```python
from build123d import *

# Parameters (mm, degrees)
F0_W     = 0.8
F0_H     = 36.4
F0_W_2   = 8.8
F0_H_2   = 1.5
F1_DEPTH = 2
F2_DEPTH = 10
F3_DEPTH = 4.15
F0_H_3   = 3.6
F4_DEPTH = 2
F5_W     = 1.5
F5_H     = 2.85
F6_DEPTH = 8.8
F0_W_3   = 28.8
F0_H_4   = 1.2
F7_DEPTH = 10


with BuildPart() as f1:
    # F0 (on Top) → F1 (new body)
    with BuildSketch(Plane.XY):
        Polygon((-15.506923, -17.20208), (-15.506923, 31.19792), (-7.006923, 31.19792), (-7.006923, 32.69792), (-17.006923, 32.69792), (-17.006923, -18.70208), (11.793077, -18.70208), (11.793077, 32.69792), (1.793077, 32.69792), (1.793077, 31.19792), (10.293077, 31.19792), (10.293077, -17.20208), align=None)
        Polygon((-7.006923, 31.19792), (-15.506923, 31.19792), (-15.506923, -17.20208), (10.293077, -17.20208), (10.293077, 31.19792), (1.793077, 31.19792), align=None)
        with Locations((-13.956923, 6.99792)):
            Rectangle(F0_W, F0_H, mode=Mode.SUBTRACT)
        Polygon((8.343077, -11.20208), (8.343077, 21.59792), (7.483077, 21.59792), (7.483077, 26.77792), (8.743077, 26.77792), (10.003077, 26.77792), (10.003077, 21.59792), (9.143077, 21.59792), (9.143077, -11.20208), align=None, mode=Mode.SUBTRACT)
        with Locations((-2.606923, 31.94792)):
            Rectangle(F0_W_2, F0_H_2)
    extrude(amount=-F1_DEPTH)

    # F0 (on Top) → F2 (join)
    with BuildSketch(Plane.XY):
        Polygon((-15.506923, -17.20208), (-15.506923, 31.19792), (-7.006923, 31.19792), (-7.006923, 32.69792), (-17.006923, 32.69792), (-17.006923, -18.70208), (11.793077, -18.70208), (11.793077, 32.69792), (1.793077, 32.69792), (1.793077, 31.19792), (10.293077, 31.19792), (10.293077, -17.20208), align=None)
    extrude(amount=F2_DEPTH)

    # F0 (on Top) → F3 (join)
    with BuildSketch(Plane.XY):
        with Locations((-2.606923, 31.94792)):
            Rectangle(F0_W_2, F0_H_2)
    extrude(amount=F3_DEPTH)

    # F0 (on Top) → F4 (cut)
    with BuildSketch(Plane.XY):
        with Locations((-13.956923, 6.99792)):
            Rectangle(F0_W, F0_H)
        with Locations((8.743077, 23.39792)):
            Rectangle(F0_W, F0_H_3)
    extrude(amount=-F4_DEPTH, mode=Mode.SUBTRACT)

    # F5 (on face) → F6 (join)
    with BuildSketch(Plane.YZ.offset(-7.006923)):
        with Locations((31.94792, 8.575)):
            Rectangle(F5_W, F5_H)
    extrude(amount=F6_DEPTH)

    # F0 (on Top) → F7 (join)
    with BuildSketch(Plane.XY):
        with Locations((-2.606923, -19.30208)):
            Rectangle(F0_W_3, F0_H_4)
    extrude(amount=F7_DEPTH)


solid = f1.part
```
The model under review builds one solid part; all positions refer to its coordinate system, in mm. A direction names the side the tool comes from. Round coordinates to 2 decimals unless told otherwise and drop trailing zeros. Write each loop counter-clockwise with the first axis right and the second up, starting at its lowest first coordinate (ties: lowest second). Pieces come first, ordered by that corner, then holes. Notation, with made-up numbers: (71.5, 10) - (75.5, 10) arc R21 ccw to (75.5, 17) - close; hole circle Ø9 at (-18, 25). An arc over 180 degrees is marked (long way). Answer as CSV lines item,"result". Start each with the question number.
(1) We need section B-B on x = -2. State the section outline as (y, z) points.
(2) Draft analysis for pull direction Y (two halves, no side actions). For faces 6 (the flat face through (-3, -19, 0)), 7 (the flat face through (-3, -18.702, -1)), 8 (the flat face through (9, 26.778, -1)), state which applies: pulls with the +Y half, pulls with the -Y half, needs draft (parallel to the pull), parting line crosses it, or undercut.
(3) We need section A-A on y = -10. State the section outline as (x, z) points, plus the area to 3 significant figures.
(4) For faces 1 (the flat face through (-3, 32, 4.15)), 2 (the flat face through (-16.5, 6.5, 10)), 3 (the flat face through (-17.007, 6, 4)), 4 (the flat face through (-14.357, 7, -1)), 5 (the flat face through (-3, 31.198, 4)), list the 3-axis set-ups (+Z, -Z, +X, -X, +Y, -Y) from which the entire face can be reached by the end or side of a thin tool; tool diameter is ignored.
(5) For pin 1 Ø1 at (x, z) = (0.5, 5) entering from +Y; pin 2 Ø6 at (x, y) = (-7.5, -4.5) entering from +Z; pin 3 Ø1.3 at (x, y) = (-5.5, -19.5) entering from -Z, all flat-tipped, find the tip position at first contact; note any pin that passes through.
(6) To check wall thickness, follow line 1 (X direction, y = 21.5, z = -1.5); line 2 (Y direction, x = -9, z = 0.25); line 3 (X direction, y = -7.5, z = 7.5). State the ranges of each line that lie inside material, in increasing order.
(7) We need section D-D on y = -16. State the section outline as (x, z) points, plus the area to 3 significant figures.
(8) We need section C-C on z = 3. State the section outline as (x, y) points.
Worked answers:
1,outline,"(-19.9, 0) - (-18.7, 0) - (-18.7, -2) - (32.7, -2) - (32.7, 4.15) - (31.2, 4.15) - (31.2, 0) - (-17.2, 0) - (-17.2, 10) - (-19.9, 10) - close; (31.2, 7.15) - (32.7, 7.15) - (32.7, 10) - (31.2, 10) - close"
2,face 6,"needs draft"
2,face 7,"pulls with the -Y half"
2,face 8,"undercut"
3,outline,"(-17.01, -2) - (-14.36, -2) - (-14.36, 0) - (-15.51, 0) - (-15.51, 10) - (-17.01, 10) - close; (-13.56, -2) - (8.34, -2) - (8.34, 0) - (-13.56, 0) - close; (9.14, -2) - (11.79, -2) - (11.79, 10) - (10.29, 10) - (10.29, 0) - (9.14, 0) - close"
3,area,"84.4 mm²"
4,face 1,"+Y"
4,face 2,"+Z, +X, -X, +Y, -Y"
4,face 3,"+Z, -Z, -X, +Y, -Y"
4,face 4,"+Z, -Z"
4,face 5,"+Z"
5,pin 1,"y = -17.2"
5,pin 2,"z = 0"
5,pin 3,"z = 0"
6,line 1,"-17.01 to -14.36, -13.56 to 8.34, 9.14 to 11.79"
6,line 2,"-19.9 to -17.2, 31.2 to 32.7"
6,line 3,"-17.01 to -15.51, 10.29 to 11.79"
7,outline,"(-17.01, -2) - (11.79, -2) - (11.79, 10) - (10.29, 10) - (10.29, 0) - (-15.51, 0) - (-15.51, 10) - (-17.01, 10) - close"
7,area,"87.6 mm²"
8,outline,"(-17.01, -19.9) - (11.79, -19.9) - (11.79, 32.7) - (-17.01, 32.7) - close; hole (-15.51, -17.2) - (10.29, -17.2) - (10.29, 31.2) - (-15.51, 31.2) - close"
